Check sheet for the drawn part. Datum: minimum x, y, z corner. Units: mm. A direction names the side the tool comes from. Round coordinates to 2 decimals unless told otherwise and drop trailing zeros. Order: outer loops, then holes, each group sorted by start corner. A loop starts at its lowest first (then second) coordinate and runs counter-clockwise, first axis right, second up.
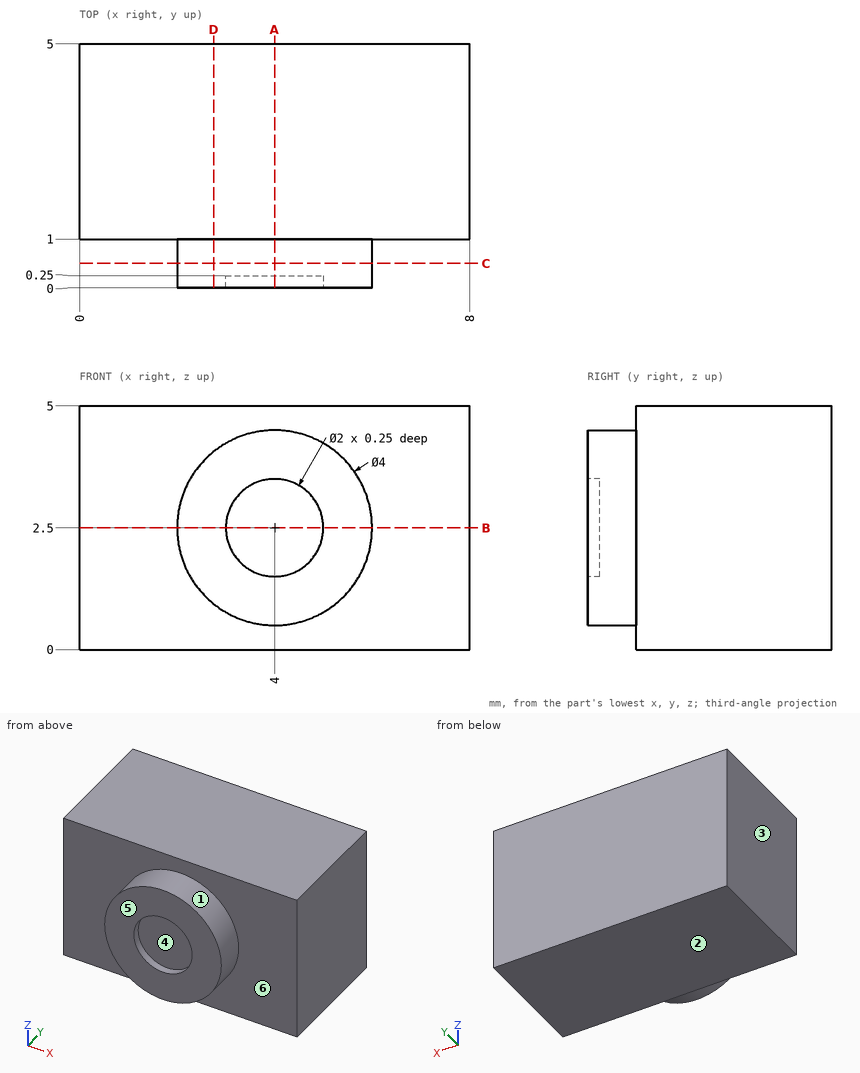
1) Sectioned sample at C-C on y = 0.5. Record the cut outline in (x, z), and give its area (3 significant figures).
2) Scan lines: line 1 (Z direction, x = 4, y = 0.1); line 2 (X direction, y = 0.15, z = 2.5); line 3 (Y direction, x = 6.75, z = 0.95). Record each from-to range of solid material in increasing order.
3) Set-up check for the marked faces 5 and 6: record each of +Z, -Z, +X, -X, +Y, -Y from which the full face is reachable in a straight line by a thin tool's end or side.
4) Sectioned sample at B-B on z = 2.5. Record the cut outline in (x, y), and give its area (3 significant figures).
5) Sectioned sample at A-A on x = 4. Record the cut outline in (y, z), and give its area (3 significant figures).
6) Draft check along X on the marked faces 1, 2, 3 and 4. Enter one of: pulls with the +X half, pulls with the -X half, needs draft (parallel to the pull), parting line crosses it, or undercut.
7) Sectioned sample at D-D on x = 2.75. Record the cut outline in (y, z), and give its area (3 significant figures).
Values found:
1. outline: circle Ø4 at (4, 2.5)
1. area: 12.6 mm2
2. line 1: z = 0.5 to 1.5, 3.5 to 4.5
2. line 2: x = 2 to 3, 5 to 6
2. line 3: y = 1 to 5
3. face 5: +Z, -Z, +X, -X, -Y
3. face 6: -Y
4. outline: (0, 1) - (2, 1) - (2, 0) - (3, 0) - (3, 0.25) - (5, 0.25) - (5, 0) - (6, 0) - (6, 1) - (8, 1) - (8, 5) - (0, 5) - close
4. area: 35.5 mm2
5. outline: (0, 0.5) - (1, 0.5) - (1, 0) - (5, 0) - (5, 5) - (1, 5) - (1, 4.5) - (0, 4.5) - (0, 3.5) - (0.25, 3.5) - (0.25, 1.5) - (0, 1.5) - close
5. area: 23.5 mm2
6. face 1: parting line crosses it
6. face 2: needs draft
6. face 3: pulls with the -X half
6. face 4: undercut
7. outline: (0, 0.94) - (1, 0.94) - (1, 0) - (5, 0) - (5, 5) - (1, 5) - (1, 4.06) - (0, 4.06) - close
7. area: 23.1 mm2
